The model under review builds one solid part; all positions refer to its coordinate system, in mm. A direction names the side the tool comes from. Round coordinates to 2 decimals unless told otherwise and drop trailing zeros. Loops run counter-clockwise (first coordinate to the right, second up) from the corner with the lowest first, then second, coordinate; pieces in that order, holes last. Notation, with made-up numbers: (-15, -33.75) -> (23, -33.75) arc R21 cw to (23, -3.75) -> close; hole circle Ø7 at (56, 5). An arc over 180 degrees is marked (long way). Use a Markdown table: item, result. Add a question column.
1) Consider section C-C on y = 75.5. Give the boundary of the cut face in (x, z).
2) Consider section A-A on x = 500. Give the boundary of the cut face in (y, z).
3) Consider section B-B on x = 466.5. Give the boundary of the cut face in (y, z), plus the area to 3 significant figures.
4) Insertion check: pin 1 (0.8 mm diameter, centred on y = 41.5, z = 0.5, fed in from -X); pin 2 (1.5 mm diameter, centred on y = 17, z = 0.5, fed in from +X); pin 3 (1.5 mm diameter, centred on x = 488.5, z = -1, fed in from -Y). Each pin has a flat end and moves straight along its axis. Give the tip position at first contact, or say it passes through.
5) For faces 1 (the flat face through (501.206, 21, 0)), 2 (the flat face through (479.233, 67.704, 0.021)), 3 (the flat face through (499, 42.073, 0)), 4 (the flat face through (504.206, 68, 0)), 5 (the flat face through (478.82, 34.36, 0.02)), list the 3-axis set-ups (+Z, -Z, +X, -X, +Y, -Y) from which the entire face can be reached by the end or side of a thin tool; tool diameter is ignored.
6) Wall thickness on probe 1 along Y at (x, z) = (500.5, -0.1); probe 2 along Y at (x, z) = (502, -0.15); probe 3 along Y at (x, z) = (487, 0.15): over which ranges is each line inside the solid? List them lowest first.
from build123d import *

# Parameters (mm, degrees)
SALIENTE_EXTRUIR1_DEPTH = 1.5


with BuildPart() as part:
    # Croquis1 → Saliente-Extruir1 (new, symmetric)
    with BuildSketch(Plane.XY):
        Polygon((484.855720511, 82.973038085), (491.215178715, 82.973038085), (501.205555648, 82.973038085), (501.205555648, 73.173108985), (504.205555648, 73.173108985), (504.205555648, 63.173108985), (501.205555648, 63.173108985), (501.205555648, 45.073108985), (497.205555648, 45.073108985), (497.205555648, 47.573108985), (494.205555648, 47.573108985), (494.205555648, 45.073108985), (493.205555648, 45.073108985), (493.205555648, 42.073108985), (494.205555648, 42.073108985), (494.205555648, 39.573108985), (497.205555648, 39.573108985), (497.205555648, 42.073108985), (501.205555648, 42.073108985), (501.205555648, 38.173108985), (504.205555648, 38.173108985), (504.205555648, 28.173108985), (501.205555648, 28.173108985), (501.205555648, 12.773108985), (494.855720505, 12.773108985), (479.205555648, 12.773108985), (468.814796849, 4.447241951), (463.814796852, 4.447241951), (465.108892077, 9.276871079), (462.2111146, 10.053328214), (464.799305049, 19.712586471), (467.697082526, 18.936129336), (471.203015891, 32.02045078), (474.824900651, 31.049969683), (474.177853039, 28.635155119), (477.075967602, 27.858607662), (477.723015214, 30.273422227), (478.664792894, 30.021073658), (479.441250029, 32.918851135), (478.499472349, 33.171199704), (479.146628347, 35.586418771), (476.248513785, 36.362966228), (475.601357786, 33.94774716), (471.979473025, 34.918228257), (476.379396799, 51.33896733), (480.001281419, 50.368486271), (479.354233806, 47.953671707), (482.252348369, 47.177124251), (482.899395981, 49.591938815), (483.841173662, 49.339590246), (484.617630796, 52.237367723), (483.675853116, 52.489716292), (484.323009115, 54.904935359), (481.424894552, 55.681482816), (480.777738553, 53.266263749), (477.155853934, 54.236744807), (480.661787289, 67.321066215), (477.764009811, 68.097523349), (480.352200261, 77.756781606), (483.249977738, 76.980324471), align=None)
    extrude(amount=SALIENTE_EXTRUIR1_DEPTH, both=True)


solid = part.part
Result set:
| question | item | result |
|---|---|---|
| 1 | outline | (479.75, -1.5) -> (501.21, -1.5) -> (501.21, 1.5) -> (479.75, 1.5) -> close |
| 2 | outline | (12.77, -1.5) -> (42.07, -1.5) -> (42.07, 1.5) -> (12.77, 1.5) -> close; (45.07, -1.5) -> (82.97, -1.5) -> (82.97, 1.5) -> (45.07, 1.5) -> close |
| 3 | outline | (4.45, -1.5) -> (19.26, -1.5) -> (19.26, 1.5) -> (4.45, 1.5) -> close |
| 3 | area | 44.4 mm2 |
| 4 | pin 1 | x = 473.64 |
| 4 | pin 2 | x = 501.21 |
| 4 | pin 3 | y = 12.77 |
| 5 | face 1 | +Z, -Z, +X, -Y |
| 5 | face 2 | +Z, -Z, -X |
| 5 | face 3 | +Z, -Z, +X |
| 5 | face 4 | +Z, -Z, +X, +Y, -Y |
| 5 | face 5 | +Z, -Z |
| 6 | probe 1 | 12.77 to 42.07, 45.07 to 82.97 |
| 6 | probe 2 | 28.17 to 38.17, 63.17 to 73.17 |
| 6 | probe 3 | 12.77 to 82.97 |
